```python
from build123d import *

# Parameters (mm, degrees)
F0_R          = 24
F0_R_2        = 17.5
F1_DEPTH      = 140
F3_DEPTH      = 24.001
F3_DEPTH_BACK = 24.001


with BuildPart() as f1:
    # F0 (on Top) → F1 (new body)
    with BuildSketch(Plane.XY):
        Circle(F0_R)
        Circle(F0_R_2, mode=Mode.SUBTRACT)
    extrude(amount=F1_DEPTH)

    # F2 (on Front) → F3 (cut, two sides)
    with BuildSketch(Plane.XZ) as f3_sk:
        with BuildLine():
            ThreePointArc((-10, 21.25), (0, 11.25), (10, 21.25))
            Line((10, 21.25), (10, 63.75))
            ThreePointArc((10, 63.75), (0, 73.75), (-10, 63.75))
            Line((-10, 63.75), (-10, 21.25))
        make_face()
    extrude(amount=-F3_DEPTH, mode=Mode.SUBTRACT)
    extrude(f3_sk.sketch, amount=F3_DEPTH_BACK, mode=Mode.SUBTRACT)


solid = f1.part
```
Can you work these out from the model? Positions are in its coordinate system, mm. A direction names the side the tool comes from. Coordinates: 2 decimals unless noted, no trailing zeros. Loops run counter-clockwise (first coordinate to the right, second up) from the corner with the lowest first, then second, coordinate; pieces in that order, holes last. Notation, with made-up numbers: (3.25, 88) - (48.25, 88) arc R33 cw to (48.25, 117) - close; hole circle Ø9 at (1, -31.75). An arc over 180 degrees is marked (long way). Use a Markdown table: item, result.
Item 1: We'd pull the mould along Z, two halves only. Please class faces 3 (the face through (-10, 18, 43)), 4 (the face through (2, -18, 140)), 5 (the face through (2, -18, 0)): released by +Z, released by -Z, zero draft, split by the parting line, or undercut.
Numbers:
| item | result |
|---|---|
| face 3 | undercut |
| face 4 | released by +Z |
| face 5 | released by -Z |
Item 2: I want a section at D-D on x = 7.5. Please give me the cut outline in (y, z).
Numbers:
| item | result |
|---|---|
| outline | (-22.8, 0) - (-15.81, 0) - (-15.81, 14.64) - (-22.8, 14.64) - close; (-22.8, 70.36) - (-15.81, 70.36) - (-15.81, 140) - (-22.8, 140) - close; (15.81, 0) - (22.8, 0) - (22.8, 14.64) - (15.81, 14.64) - close; (15.81, 70.36) - (22.8, 70.36) - (22.8, 140) - (15.81, 140) - close |
Item 3: Will these pins go through, and if not, where does the flat tip stop? pin 1 (4 mm diameter, centred on x = -15, z = 33.5, fed in from -Y); pin 2 (12 mm diameter, centred on y = 10, z = 107, fed in from -X); pin 3 (4 mm diameter, centred on y = 4, z = 80, fed in from -X); pin 4 (2 mm diameter, centred on x = 14, y = -8, fed in from -Z).
Numbers:
| item | result |
|---|---|
| pin 1 | stops at y = -20.17 |
| pin 2 | stops at x = -23.66 |
| pin 3 | stops at x = -23.92 |
| pin 4 | passes through |
Item 4: I want a section at A-A on y = 0. Please give me the cut outline in (x, z).
Numbers:
| item | result |
|---|---|
| outline | (-24, 0) - (-17.5, 0) - (-17.5, 140) - (-24, 140) - close; (17.5, 0) - (24, 0) - (24, 140) - (17.5, 140) - close |
Item 5: I want a section at B-B on z = 31.5. Please give me the cut outline in (x, y).
Numbers:
| item | result |
|---|---|
| outline | (-10, -21.82) - (-10, -14.36) arc R17.5 cw to (-10, 14.36) - (-10, 21.82) arc R24 ccw to start; (10, -21.82) arc R24 ccw to (10, 21.82) - (10, 14.36) arc R17.5 cw to (10, -14.36) - close |
Item 6: If I drill on probe 1 along Y at (x, z) = (0, 94); probe 2 along Y at (x, z) = (-13.5, 19); probe 3 along X at (y, z) = (20.5, 17.5), over which ranges is the centre line in solid material (lowest first)? Write a range as from..to.
Numbers:
| item | result |
|---|---|
| probe 1 | y = -24..-17.5, 17.5..24 |
| probe 2 | y = -19.84..-11.14, 11.14..19.84 |
| probe 3 | x = -12.48..-9.27, 9.27..12.48 |
Item 7: I want a section at C-C on x = 0. Please give me the cut outline in (y, z), and give its area (3 significant figures).
Numbers:
| item | result |
|---|---|
| outline | (-24, 0) - (-17.5, 0) - (-17.5, 11.25) - (-24, 11.25) - close; (-24, 73.75) - (-17.5, 73.75) - (-17.5, 140) - (-24, 140) - close; (17.5, 0) - (24, 0) - (24, 11.25) - (17.5, 11.25) - close; (17.5, 73.75) - (24, 73.75) - (24, 140) - (17.5, 140) - close |
| area | 1,010 mm2 |
Item 8: For faces 1 (the face through (-10, -18, 43)), 2 (the face through (-12.898, 11.827, 69.02)), which set-ups out of +Z, -Z, +X, -X, +Y, -Y let a thin tool reach every point of the face, with its end or its side?
Numbers:
| item | result |
|---|---|
| face 1 | +Y, -Y |
| face 2 | +Z, -Z |
